Here's how the part is built. I have some questions about the finished solid (model axes, mm). A direction names the side the tool comes from. Coordinates: 2 decimals unless noted, no trailing zeros. Write each loop counter-clockwise with the first axis right and the second up, starting at its lowest first coordinate (ties: lowest second). Pieces come first, ordered by that corner, then holes.
```python
from build123d import *

# Parameters (mm, degrees)
F2_R     = 4
F3_DEPTH = 150.001


with BuildPart() as f1:
    # F0 (on Front) → F1 (revolve)
    with BuildSketch(Plane.XZ):
        with BuildLine():
            Line((-54.5, 0), (0, 0))
            Line((0, 0), (0, 10))
            Line((0, 10), (-40, 10))
            ThreePointArc((-40, 10), (-43.535534, 11.464466), (-45, 15))
            Line((-45, 15), (-45, 135))
            ThreePointArc((-45, 135), (-43.535534, 138.535534), (-40, 140))
            Line((-40, 140), (0, 140))
            Line((0, 140), (0, 150))
            Line((0, 150), (-54.5, 150))
            ThreePointArc((-54.5, 150), (-54.853553, 149.853553), (-55, 149.5))
            Line((-55, 149.5), (-55, 0.5))
            ThreePointArc((-55, 0.5), (-54.853553, 0.146447), (-54.5, 0))
        make_face()
    revolve(axis=Axis((0, 0, 48.276713), (0, 0, 1)))

    # F2 (on face) → F3 (cut, through all)
    with BuildSketch(Plane.XY.offset(150)):
        with Locations((30, 0)):
            Circle(F2_R)
        with Locations((0, 30)):
            Circle(F2_R)
        with Locations((-30, 0)):
            Circle(F2_R)
        with Locations((0, -30)):
            Circle(F2_R)
    extrude(amount=-F3_DEPTH, mode=Mode.SUBTRACT)


solid = f1.part
```
1) Will these pins go through, and if not, where does the flat tip stop? pin 1 (2 mm diameter, centred on x = -17, z = 87.5, fed in from -Y); pin 2 (12 mm diameter, centred on x = 32, z = 65, fed in from +Y); pin 3 (10 mm diameter, centred on y = 34.5, z = 122.5, fed in from -X).
Values follow:
pin 1: stops at y = -52.62
pin 2: stops at y = 48.47
pin 3: stops at x = -46.42
2) Imagine slicing it at A-A on x = 0. Count the separate pieces of the cut face and the enclosed holes in it, then the cut area to 3 significant figures.
Values follow:
separate pieces: 4
enclosed holes: 0
area: 4,500 mm2
3) We'd pull the mould along Z, two halves only. Please class faces 3 (the face through (26.8, -2.4, 5.1)), 4 (the face through (-20.765, 39.923, 75.84)), 5 (the face through (1, -1, 0)): pulls with the +Z half, pulls with the -Z half, needs draft (parallel to the pull), parting line crosses it, or undercut.
Values follow:
face 3: needs draft
face 4: undercut
face 5: pulls with the -Z half
4) I need wall thicknesses on probe 1 along Z at (x, y) = (-21.5, -1); probe 2 along X at (y, z) = (1, 88.5); probe 3 along Y at (x, z) = (0, 94.5). Which ranges of each line are inside material? Lowest first, please.
Values follow:
probe 1: z = 0 to 10, 140 to 150
probe 2: x = -54.99 to -44.99, 44.99 to 54.99
probe 3: y = -55 to -45, 45 to 55
5) On a 3-axis mill with a long thin cutter (end or side, diameter ignored), from which of +Z, -Z, +X, -X, +Y, -Y can I reach the whole of each face in a straight line? I mean faces 1 (the face through (-0.521, -26.034, 145.07)), 2 (the face through (1, -1, 140)). Say none if no direction works.
Values follow:
face 1: +Z, -Z
face 2: none
6) Imagine slicing it at D-D on z = 35.5. Please give me the cut outline in (x, y), then the cut area to 3 significant figures.
Values follow:
outline: circle Ø110 at (0, 0); hole circle Ø90 at (0, 0)
area: 3,140 mm2
7) Imagine slicing it at C-C on z = 12. Please give me the cut outline in (x, y), then the cut area to 3 significant figures.
Values follow:
outline: circle Ø110 at (0, 0); hole circle Ø88 at (0, 0)
area: 3,420 mm2
